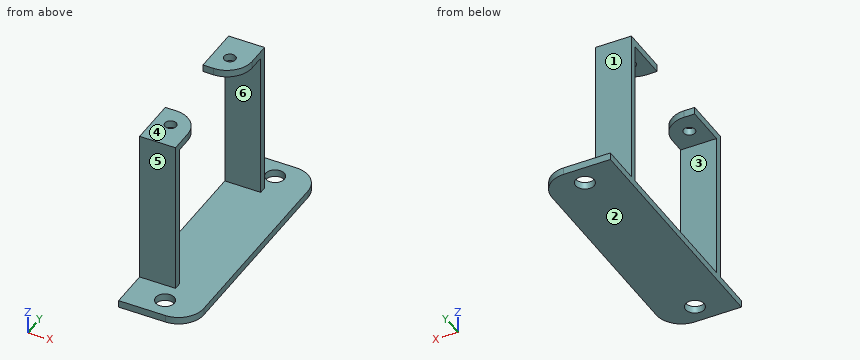
from build123d import *

# Parameters (mm, degrees)
F0_W     = 10
F0_H     = 42.6
F1_DEPTH = 2
F0_H_2   = 2
F2_DEPTH = 43.2
F3_W     = 10
F3_H     = 2
F3_H_2   = 13.45
F3_H_3   = 11.45
F4_DEPTH = 2
F5_D     = 3.2
F5_DEPTH = 2.001
F6_D     = 5.2
F7_R     = 7


with BuildPart() as f1:
    # F0 (on Top) → F1 (new body)
    with BuildSketch(Plane.XY):
        with Locations((-61.0561398208, -14.4174070306)):
            Rectangle(F0_W, F0_H)
        Polygon((-61.0561398208, -48.7174070306), (-51.0561398208, -48.7174070306), (-51.0561398208, -37.7174070306), (-56.0561398208, -37.7174070306), (-66.0561398208, -37.7174070306), (-66.0561398208, -48.7174070306), align=None)
        Polygon((-51.0561398208, 19.8825929694), (-61.0561398208, 19.8825929694), (-66.0561398208, 19.8825929694), (-66.0561398208, 8.8825929694), (-56.0561398208, 8.8825929694), (-51.0561398208, 8.8825929694), align=None)
        Polygon((-46.0561398208, 19.8825929694), (-51.0561398208, 19.8825929694), (-51.0561398208, 8.8825929694), (-56.0561398208, 8.8825929694), (-56.0561398208, 6.8825929694), (-56.0561398208, -35.7174070306), (-56.0561398208, -37.7174070306), (-51.0561398208, -37.7174070306), (-51.0561398208, -48.7174070306), (-46.0561398208, -48.7174070306), align=None)
    extrude(amount=F1_DEPTH)

    # F0 (on Top) → F2 (join)
    with BuildSketch(Plane.XY):
        with Locations((-61.0561398208, -36.7174070306)):
            Rectangle(F0_W, F0_H_2)
        with Locations((-61.0561398208, 7.8825929694)):
            Rectangle(F0_W, F0_H_2)
    extrude(amount=F2_DEPTH)

    # F3 (on face) → F4 (join)
    with BuildSketch(Plane.XY.offset(43.2)):
        with Locations((-61.0561398208, -36.7174070306)):
            Rectangle(F3_W, F3_H)
        with Locations((-61.0561398208, 2.1575929694)):
            Rectangle(F3_W, F3_H_2)
        with Locations((-61.0561398208, -29.9924070306)):
            Rectangle(F3_W, F3_H_3)
    extrude(amount=F4_DEPTH)

    # F5 (through all, one way)
    with BuildSketch(Plane(origin=(0, 0, 43.2), x_dir=(1, 0, 0), z_dir=(0, 0, -1))):
        with Locations((-61.5561398208, -1.0825929694), (-61.5561398208, 29.9174070306)):
            Circle(F5_D / 2)
    extrude(amount=-F5_DEPTH, mode=Mode.SUBTRACT)

    # F6 (through all)
    with Locations(Plane(origin=(0, 0, 0), x_dir=(1, 0, 0), z_dir=(0, 0, -1))):
        with Locations((-56.0561398208, -14.3825929694), (-56.0561398208, 43.2174070306)):
            Hole(F6_D / 2)

    # F7
    f7_edges = [f1.edges().sort_by_distance(p)[0] for p in [
        (-56.05614, -4.567407, 44.2),
        (-56.05614, -24.267407, 44.2),
        (-46.05614, 19.882593, 1),
        (-46.05614, -48.717407, 1),
    ]]
    fillet(f7_edges, radius=F7_R)


solid = f1.part
Could you check a few things on this model? Use its own coordinates, in mm. Face numbers are marked on the shaded views. A direction names the side the tool comes from. Coordinates: 2 decimals unless noted, no trailing zeros. Write each loop counter-clockwise with the first axis right and the second up, starting at its lowest first coordinate (ties: lowest second). Pieces come first, ordered by that corner, then holes. Notation, with made-up numbers: (52, -32) - (105, -32) arc R12 ccw to (105, -28) - close; hole circle Ø2 at (73.25, -35.5). An arc over 180 degrees is marked (long way). Put each result on its own line as item: value. Start each with the question number.
Q1. I want a section at B-B on x = -57. Write out the boundary of the cut face in (y, z), plus the area to 3 significant figures.
Q2. I want a section at A-A on z = 7. Write out the boundary of the cut face in (x, y), plus the area to 3 significant figures.
Q3. I'm going to push flat-ended pins straight in: P1, Ø3, axis at x = -55, y = -28, coming from the +Z side; P2, Ø3, axis at y = -40.5, z = 6, coming from the -X side; P3, Ø1, axis at x = -64.5, z = 44, coming from the +Y side; P4, Ø7, axis at y = -36, z = 27, coming from the +X side. Where does each tip first touch, or does it pass through?
Q4. Which directions (+Z, -Z, +X, -X, +Y, -Y) give clear straight access to the entire face, cutting with the end or side of a thin tool? Please do the marked faces 4, 5 and 6.
Q5. Thinking about a two-plate mould opening in Z: for the marked faces 1, 2 and 3, which applies, pulls with the +Z half, pulls with the -Z half, needs draft (parallel to the pull), parting line crosses it, or undercut?
Q6. Please list where these lines run through material, in increasing order: L1, parallel to Y at x = -60.75, z = 5; L2, parallel to Z at x = -62.75, y = 4; L3, parallel to Z at x = -63.5, y = -24.
Q7. I want a section at D-D on y = -25.5. Write out the boundary of the cut face in (x, z), plus the area to 3 significant figures.
Q8. I want a section at C-C on x = -64.5. Write out the boundary of the cut face in (y, z).
Checks:
1. outline: (-48.72, 0) - (-45.64, 0) - (-45.64, 2) - (-48.72, 2) - close; (-40.79, 0) - (11.96, 0) - (11.96, 2) - (8.88, 2) - (8.88, 45.2) - (-1.08, 45.2) - (-1.08, 43.2) - (6.88, 43.2) - (6.88, 2) - (-35.72, 2) - (-35.72, 43.2) - (-27.76, 43.2) - (-27.76, 45.2) - (-37.72, 45.2) - (-37.72, 2) - (-40.79, 2) - close; (16.81, 0) - (19.88, 0) - (19.88, 2) - (16.81, 2) - close
1. area: 322 mm²
2. outline: (-66.06, -37.72) - (-56.06, -37.72) - (-56.06, -35.72) - (-66.06, -35.72) - close; (-66.06, 6.88) - (-56.06, 6.88) - (-56.06, 8.88) - (-66.06, 8.88) - close
2. area: 40.0 mm²
3. P1: z = 2
3. P2: through
3. P3: y = 8.88
3. P4: x = -56.06
4. face 4: +Z, +X, -X, +Y, -Y
4. face 5: +Z, +X, -X, -Y
4. face 6: +X, -X
5. face 1: needs draft
5. face 2: pulls with the -Z half
5. face 3: undercut
6. L1: -37.72 to -35.72, 6.88 to 8.88
6. L2: 0 to 2, 43.2 to 45.2
6. L3: 0 to 2
7. outline: (-66.06, 0) - (-46.06, 0) - (-46.06, 2) - (-66.06, 2) - close; (-66.06, 43.2) - (-59.09, 43.2) - (-59.09, 45.2) - (-66.06, 45.2) - close
7. area: 53.9 mm²
8. outline: (-48.72, 0) - (19.88, 0) - (19.88, 2) - (8.88, 2) - (8.88, 45.2) - (-4.57, 45.2) - (-4.57, 43.2) - (6.88, 43.2) - (6.88, 2) - (-35.72, 2) - (-35.72, 43.2) - (-24.27, 43.2) - (-24.27, 45.2) - (-37.72, 45.2) - (-37.72, 2) - (-48.72, 2) - close
